Read the model definition and answer for the solid it produces. Units are mm, in the model's axes. A direction names the side the tool comes from. Give positions to 0.01 mm unless a question says otherwise; leave off trailing zeros. Write each loop counter-clockwise with the first axis right and the second up, starting at its lowest first coordinate (ties: lowest second). Pieces come first, ordered by that corner, then holes. Notation, with made-up numbers: (6.5, 85) - (27.5, 85) arc R21 ccw to (27.5, 101) - close; hole circle Ø10 at (36.5, 35.25). An arc over 180 degrees is marked (long way). Answer as a JSON object with one key per item and string values. Group by question number.
Autodesk Inventor part; units mm, degrees
ref_plane "YZ Plane" through (0, 0, 0) normal (1, 0, 0) x (0, 1, 0)
ref_plane "XZ Plane" through (0, 0, 0) normal (0, 1, 0) x (-1, 0, 0)
ref_plane "XY Plane" through (0, 0, 0) normal (0, 0, 1) x (1, 0, 0)
sketch "Эскиз1" plane through (0, 0, 0) normal (0, 1, 0) x (-1, 0, 0)
  line L0 (0, 25.8601) -> (0, -22.7313) construction
  arc A0 (8.1832, 2.5181) -> (8.1832, 6.1819) centre (6, 4.35) ccw construction
  line L1 (6, 4.35) -> (8.85, 4.35) construction
  line L2 (6, 4.35) -> (8.1832, 2.5181) construction
  line L3 (6, 4.35) -> (8.1832, 6.1819) construction
  arc A1 (6, 8.7) -> (6, 0) centre (6, 4.35) ccw construction
  line L4 (6, 0) -> (0, 0)
  line L5 (6, 8.7) -> (0, 8.7)
  arc A2 (9.3323, 7.1461) -> (6, 8.7) centre (6, 4.35) ccw
  arc A3 (9.3323, 1.5539) -> (9.3323, 7.1461) centre (6, 4.35) ccw construction
  arc A4 (6, 0) -> (9.3323, 1.5539) centre (6, 4.35) ccw
  line L6 (8.1832, 2.5181) -> (9.3323, 1.5539)
  line L7 (8.1832, 6.1819) -> (9.3323, 7.1461)
  arc A5 (8.1832, 6.1819) -> (8.1832, 2.5181) centre (6, 4.35) ccw
  line L8 (0, 0) -> (0, 8.7)
  line L9 (-3, 11.85) -> (0, 11.85)
  line L10 (0, 11.85) -> (0, -3.15)
  line L11 (0, -3.15) -> (-3, -3.15)
  line L12 (-3, -3.15) -> (-3, 11.85)
  point P0 (0, 4.35)
  point P1 (0, 0)
  point P2 (0, 8.7)
  dimension "d0" = 5.7
  dimension "d1" = 80
  dimension "d3" = 6
  dimension "d6" = 15
  dimension "d7" = 3
  dimension "d12" = 1.5
  dimension "d15" = 80
extrude "Выдавливание1" add sketch "Эскиз1" along normal blind 8 contours L4 L8 L5 A2 L7 A5 L6 A4
extrude "Выдавливание2" add sketch "Эскиз1" along normal blind 10 contours L10 L11 L12 L9 L8
fillet "Сопряжение3" radius 0.7 2 edges at (-8.1832, 4, 2.5181) (-8.1832, 4, 6.1819)
fillet "Сопряжение4" radius 0.9 2 edges at (-9.3323, 4, 1.5539) (-9.3323, 4, 7.1461)
properties part number "stand_mount_example"
1) Find section D-D, the plane z = 1. Write down the section's boundary in (x, y), and give its area (3 significant figures).
2) Find section A-A, the plane z = 4.35. Write down the section's boundary in (x, y), and give its area (3 significant figures).
3) Which of the six approach directions +Z, -Z, +X, -X, +Y, -Y give full straight-line access (tool end or side, diameter ignored) to faces 1 (the cylindrical face through (-8.231, 4.056, 2.277)), 2 (the flat face through (-2, 8, 4)), 3 (the cylindrical face through (-7.3, 3.9, 8.5)), 4 (the flat face through (-3, 4, 0)), 5 (the flat face through (2, 5, 11.85))?
4) Find section C-C, the plane x = -1. Write down the section's boundary in (y, z), and give its area (3 significant figures).
5) Flat-ended cylindrical pins translate along their axes: pin 1 Ø2 at (x, y) = (-6.5, 8.5) entering from -Z; pin 2 Ø2 at (x, z) = (-3, 6) entering from +Y; pin 3 Ø1.8 at (x, y) = (-2, 2.5) entering from +Z. Find the tip coordinate at first contact, or state that the pin passes through.
6) Find section B-B, the plane y = 4.5. Write down the section's boundary in (x, z), and give its area (3 significant figures).
7) Find the intervals of material crossed by line 1 (Z direction, x = -6, y = 5); line 2 (X direction, y = 2, z = 4.35); line 3 (Y direction, x = -3, z = 0.25), in increasing order. Write a range as [from, to].
8) For a pull along Z with two mould halves and no side action, classify faces 6 (the flat face through (1, 5, -3.15)), 7 (the flat face through (-3, 4, 8.7)), 8 (the flat face through (3, 5, 4)), 9 (the cylindrical face through (-8.218, 4.056, 6.423)) as released by +Z, released by -Z, zero draft, split by the parting line, or undercut.
Values follow:
{
 "1": {"outline": "(-8.71, 0) - (3, 0) - (3, 10) - (0, 10) - (0, 8) - (-8.71, 8) - close", "area": "99.7 mm2"},
 "2": {"outline": "(-3.15, 0) - (3, 0) - (3, 10) - (0, 10) - (0, 8) - (-3.15, 8) - close", "area": "55.2 mm2"},
 "3": {"face 1": "+Y, -Y", "face 2": "+Z, -Z, -X, +Y", "face 3": "+Z, -X, +Y, -Y", "face 4": "-Z, -X, +Y, -Y", "face 5": "+Z, +X, -X, +Y, -Y"},
 "4": {"outline": "(0, 0) - (8, 0) - (8, 8.7) - (0, 8.7) - close", "area": "69.6 mm2"},
 "5": {"pin 1": "stops at z = 0", "pin 2": "stops at y = 8", "pin 3": "stops at z = 8.7"},
 "6": {"outline": "(-8.67, 2.11) arc R0.9 ccw to (-8.5, 0.79) arc R4.35 ccw to (-6, 0) - (0, 0) - (0, -3.15) - (3, -3.15) - (3, 11.85) - (0, 11.85) - (0, 8.7) - (-6, 8.7) arc R4.35 ccw to (-8.5, 7.91) arc R0.9 ccw to (-8.67, 6.59) arc R0.7 ccw to (-7.78, 6.58) arc R2.85 cw (long way) to (-7.78, 2.12) arc R0.7 ccw to start", "area": "93.2 mm2"},
 "7": {"line 1": "z = [0, 1.5], [7.2, 8.7]", "line 2": "x = [-3.15, 3]", "line 3": "y = [0, 8]"},
 "8": {"face 6": "released by -Z", "face 7": "released by +Z", "face 8": "zero draft", "face 9": "undercut"}
}
